from build123d import *

# Parameters (mm, degrees)
SKETCH1_R           = 21.5
SKETCH1_R_2         = 1.5
BOSS_EXTRUDE1_DEPTH = 2


with BuildPart() as part:
    # Sketch1 → Boss-Extrude1 (new body)
    with BuildSketch(Plane.XY):
        Circle(SKETCH1_R)
        Circle(SKETCH1_R_2, mode=Mode.SUBTRACT)
        Polygon((18, 2.886751346), (13, 5.773502692), (8, 2.886751346), (8, -2.886751346), (13, -5.773502692), (18, -2.886751346), align=None, mode=Mode.SUBTRACT)
    extrude(amount=BOSS_EXTRUDE1_DEPTH)


solid = part.part
Verification items for the finished model (mm, model axes). A direction names the side the tool comes from. Give positions to 0.01 mm unless a question says otherwise; leave off trailing zeros. Write each loop counter-clockwise with the first axis right and the second up, starting at its lowest first coordinate (ties: lowest second). Pieces come first, ordered by that corner, then holes. Notation, with made-up numbers: M 88,17 L 131,17 A18 ccw 131,23 Z; hole C 37.5,31.5 d1. An arc over 180 degrees is marked long. Put each result on its own line as item: value. Start each with the question number.
1. Go/stop test with flat-tipped pins: pin 1 Ø1 at (x, z) = (7.5, 0.5) entering from +Y; pin 2 Ø1.5 at (x, y) = (-16, 14) entering from -Z; pin 3 Ø1 at (y, z) = (-3, 0.5) entering from +X; pin 4 Ø0.6 at (y, z) = (0.5, 1) entering from +X. Record where each tip stops, or that it passes through.
2. Section check D-D (y = 4.5). Record the cut outline in (x, z), and give its area (3 significant figures).
3. Section check A-A (x = 0). Record the cut outline in (y, z).
4. Scan lines: line 1 along Y through (x, z) = (0, 1.3); line 2 along Y through (x, z) = (12, 0.3); line 3 along X through (y, z) = (-4, 0.4). Record each from-to range of solid material in increasing order. Write a range as [from, to].
5. Section check C-C (y = 0). Record the cut outline in (x, z).
6. Section check B-B (z = 1.6). Record the cut outline in (x, y).
7. Draft check along Y on faces 3 (the face through (0, -4, 2)), 4 (the face through (-2.799, 21.317, 0.986)), 5 (the face through (10.535, 4.35, 0.986)). Enter one of: +Y half, -Y half, draft (parallel to the pull), parting line (faces both ways), or undercut.
8. Set-up check for faces 1 (the face through (0, -4, 0)), 2 (the face through (15.535, 4.31, 0.986)): record each of +Z, -Z, +X, -X, +Y, -Y from which the full face is reachable in a straight line by a thin tool's end or side.
Answer list:
1. pin 1: y = 20.33
1. pin 2: z = 0
1. pin 3: x = 21.35
1. pin 4: x = 21.5
2. outline: M -21.02,0 L 10.79,0 L 10.79,2 L -21.02,2 Z; M 15.21,0 L 21.02,0 L 21.02,2 L 15.21,2 Z
2. area: 75.3 mm2
3. outline: M -21.5,0 L -1.5,0 L -1.5,2 L -21.5,2 Z; M 1.5,0 L 21.5,0 L 21.5,2 L 1.5,2 Z
4. line 1: [-21.5, -1.5], [1.5, 21.5]
4. line 2: [-17.84, -5.2], [5.2, 17.84]
4. line 3: [-21.12, 9.93], [16.07, 21.12]
5. outline: M -21.5,0 L -1.5,0 L -1.5,2 L -21.5,2 Z; M 1.5,0 L 8,0 L 8,2 L 1.5,2 Z; M 18,0 L 21.5,0 L 21.5,2 L 18,2 Z
6. outline: C 0,0 d43; hole C 0,0 d3; hole M 8,-2.89 L 13,-5.77 L 18,-2.89 L 18,2.89 L 13,5.77 L 8,2.89 Z
7. face 3: draft
7. face 4: parting line
7. face 5: undercut
8. face 1: -Z, +X, -X, +Y, -Y
8. face 2: +Z, -Z
